Design review of the part built by this model. Coordinates are the model's own, in mm. Face numbers are marked on the shaded views. A direction names the side the tool comes from. Give positions to 0.01 mm unless a question says otherwise; leave off trailing zeros. Loops run counter-clockwise (first coordinate to the right, second up) from the corner with the lowest first, then second, coordinate; pieces in that order, holes last. Notation, with made-up numbers: M -30,53.5 L 0,53.5 A21 cw 0,82.5 Z; hole C -11,35 d1. An arc over 180 degrees is marked long. Use a Markdown table: item, result. Add a question column.
(1) For probe 1 along Z at (x, y) = (-14.25, 0); probe 2 along Z at (x, y) = (-10, 0); probe 3 along Z at (x, y) = (-35.5, 0), list the stretches that pass through material, from the lowest coordinate up.
(2) Add section D-D, the plane x = -34.5. State how many separate pieces and enclosed holes the cut face has, then the cut area to 3 significant figures.
(3) For the marked faces 4, 5, 6, 7 and 8, list the 3-axis set-ups (+Z, -Z, +X, -X, +Y, -Y) from which the entire face can be reached by the end or side of a thin tool; tool diameter is ignored.
(4) Add section B-B, the plane z = -52. Give the boundary of the cut face in (x, y).
(5) Draft analysis for pull direction Y (two halves, no side actions). For the marked faces 1, 2 and 3, state which applies: pulls with the +Y half, pulls with the -Y half, needs draft (parallel to the pull), parting line crosses it, or undercut.
(6) Insertion check: pin 1 Ø1 at (x, y) = (-9.5, -6.5) entering from -Z; pin 2 Ø10 at (x, z) = (-67.5, -26.5) entering from +Y; pin 3 Ø5 at (y, z) = (4.5, -3.5) entering from -X. Each pin has a flat end and moves straight along its axis. Give the tip position at first contact, or say it passes through.
```python
from build123d import *

# Parameters (mm, degrees)
F0_R     = 20
F0_R_2   = 10
F4_R     = 30
F4_R_2   = 20
F5_DEPTH = 10
F7_R     = 30
F7_R_2   = 20
F8_DEPTH = 10


with BuildPart() as f2:
    # F2: sweep along a path in F1
    with BuildLine(Plane.XZ) as f2_path:
        Line((0, 0), (-20, 0))
        ThreePointArc((-20, 0), (-48.2842712475, -11.7157287525), (-60, -40))
        Line((-60, -40), (-60, -60))
    # F0 (on Right) → F2 (sweep)
    with BuildSketch(Plane.YZ):
        Circle(F0_R)
        Circle(F0_R_2, mode=Mode.SUBTRACT)
    sweep(path=f2_path.line)

    # F4 (on offset) → F5 (join)
    with BuildSketch(Plane.YZ.offset(-3)):
        Circle(F4_R)
        Circle(F4_R_2, mode=Mode.SUBTRACT)
    extrude(amount=-F5_DEPTH)

    # F7 (on offset) → F8 (join)
    with BuildSketch(Plane(origin=(0, 0, -57), x_dir=(1, 0, 0), z_dir=(0, 0, -1))):
        with Locations((-60, 0)):
            Circle(F7_R)
        with Locations((-60, 0)):
            Circle(F7_R_2, mode=Mode.SUBTRACT)
    extrude(amount=-F8_DEPTH)


solid = f2.part
```
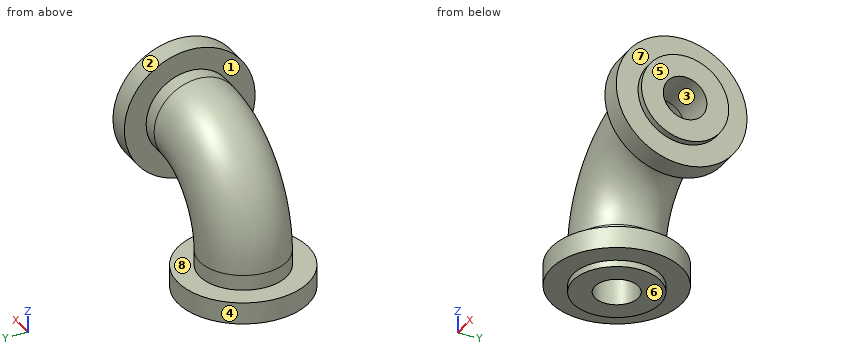
Established:
| question | item | result |
|---|---|---|
| 1 | probe 1 | -20 to -10, 10 to 20 |
| 1 | probe 2 | -30 to -10, 10 to 30 |
| 1 | probe 3 | -57 to -47, -27.36 to -14.31, 7.54 to 17.96 |
| 2 | separate pieces | 2 |
| 2 | enclosed holes | 1 |
| 2 | area | 1,360 mm^2 |
| 3 | face 4 | -Z |
| 3 | face 5 | +Z, -Z, +X, +Y, -Y |
| 3 | face 6 | -Z, +X, -X, +Y, -Y |
| 3 | face 7 | +X |
| 3 | face 8 | none |
| 4 | outline | C -60,0 d60; hole C -60,0 d20 |
| 5 | face 1 | needs draft |
| 5 | face 2 | parting line crosses it |
| 5 | face 3 | undercut |
| 6 | pin 1 | z = -29.39 |
| 6 | pin 2 | y = 19.51 |
| 6 | pin 3 | x = -68.93 |
